Autodesk Inventor part; units mm, degrees
ref_plane "YZ Plane" through (0, 0, 0) normal (1, 0, 0) x (0, 1, 0)
ref_plane "XZ Plane" through (0, 0, 0) normal (0, 1, 0) x (-1, 0, 0)
ref_plane "XY Plane" through (0, 0, 0) normal (0, 0, 1) x (1, 0, 0)
sketch "スケッチ1" plane through (0, 0, 0) normal (0, 0, 1) x (1, 0, 0)
  line L0 (12.35, 15.25) -> (9.34, 15.25)
  line L1 (-15.25, 12.35) -> (-15.25, -12.35)
  line L2 (-12.35, -15.25) -> (-1.66, -15.25)
  line L3 (15.25, -12.35) -> (15.25, 12.35)
  line L4 (-0.66, 6.75) -> (8.34, 6.75)
  line L5 (9.34, 7.75) -> (9.34, 15.25)
  line L6 (-0.66, -6.75) -> (8.34, -6.75)
  line L7 (9.34, -7.75) -> (9.34, -15.25)
  line L8 (9.34, 15.25) -> (-1.66, 15.25) construction
  line L9 (-1.66, 15.25) -> (-12.35, 15.25)
  line L10 (9.34, -15.25) -> (12.35, -15.25)
  line L11 (-1.66, -15.25) -> (9.34, -15.25) construction
  line L12 (-1.66, 15.25) -> (-1.66, 7.75)
  line L13 (-1.66, -15.25) -> (-1.66, -7.75)
  arc A0 (15.25, 12.35) -> (12.35, 15.25) centre (12.35, 12.35) ccw
  arc A1 (12.35, -15.25) -> (15.25, -12.35) centre (12.35, -12.35) ccw
  arc A2 (-15.25, -12.35) -> (-12.35, -15.25) centre (-12.35, -12.35) ccw
  arc A3 (-12.35, 15.25) -> (-15.25, 12.35) centre (-12.35, 12.35) ccw
  arc A4 (-1.66, 7.75) -> (-0.66, 6.75) centre (-0.66, 7.75) ccw
  arc A5 (8.34, 6.75) -> (9.34, 7.75) centre (8.34, 7.75) ccw
  arc A6 (9.34, -7.75) -> (8.34, -6.75) centre (8.34, -7.75) ccw
  arc A7 (-0.66, -6.75) -> (-1.66, -7.75) centre (-0.66, -7.75) ccw
  line L14 (0, 0) -> (0, -35.1049) construction
  line L15 (0, 0) -> (30.4007, 0) construction
  line L16 (3.84, -9) -> (3.84, -1.2529) construction
  arc A8 (15.35, 12.35) -> (12.35, 15.35) centre (12.35, 12.35) ccw construction
  dimension "d0" = 2.9
  dimension "d1" = 1
  dimension "d14" = 8.5
  dimension "d15" = 11
  dimension "d16" = 3.84
  dimension "d17" = 8.5
  dimension "d21" = 3
extrude "押し出し1" add sketch "スケッチ1" along normal blind 4
hole "穴1" at (12.35, 12.35, 0) at (12.35, -12.35, 0) at (-12.35, -12.35, 0) at (-12.35, 12.35, 0) direction (0, 0, 1) diameter 2.1 end through all
chamfer "面取り1" distance 0.25 angle 45 4 edges at (9.34, 15.25, 2) (-1.66, 15.25, 2) (-1.66, -15.25, 2) (9.34, -15.25, 2)
properties part number "QUIKS_SINGLE_COVER"
Source: CAD feature listing. Evaluate the final solid. Frame: model axes, mm. A direction names the side the tool comes from. Coordinates: 2 decimals unless noted, no trailing zeros. Loops run counter-clockwise (first coordinate to the right, second up) from the corner with the lowest first, then second, coordinate; pieces in that order, holes last. Notation, with made-up numbers: M 87,-4.5 L 125,-4.5 A26 ccw 125,16.5 Z; hole C 49.25,-38 d7. An arc over 180 degrees is marked long. Answer in a Markdown table with one row per item.
Q1. Section B-B on x = 2. Return the cut outline in (y, z), plus the area to 3 significant figures.
Answers below:
| item | result |
|---|---|
| outline | M -6.75,0 L 6.75,0 L 6.75,4 L -6.75,4 Z |
| area | 54.0 mm^2 |
Q2. Section A-A on z = 0.6. Return the cut outline in (x, y).
Answers below:
| item | result |
|---|---|
| outline | M -15.25,-12.35 A2.9 ccw -12.35,-15.25 L -1.91,-15.25 L -1.66,-15 L -1.66,-7.75 A1 cw -0.66,-6.75 L 8.34,-6.75 A1 cw 9.34,-7.75 L 9.34,-15 L 9.59,-15.25 L 12.35,-15.25 A2.9 ccw 15.25,-12.35 L 15.25,12.35 A2.9 ccw 12.35,15.25 L 9.59,15.25 L 9.34,15 L 9.34,7.75 A1 cw 8.34,6.75 L -0.66,6.75 A1 cw -1.66,7.75 L -1.66,15 L -1.91,15.25 L -12.35,15.25 A2.9 ccw -15.25,12.35 Z; hole C -12.35,-12.35 d2.1; hole C -12.35,12.35 d2.1; hole C 12.35,-12.35 d2.1; hole C 12.35,12.35 d2.1 |
Q3. Draft query along X for faces 4 (the flat face through (-7, -15.25, 2)), 5 (the flat face through (-15.25, 0, 2)), 6 (the cylindrical face through (12.99, -13.18, 2.03)). Return one class per face: pulls with the +X half, pulls with the -X half, needs draft (parallel to the pull), parting line crosses it, or undercut.
Answers below:
| item | result |
|---|---|
| face 4 | needs draft |
| face 5 | pulls with the -X half |
| face 6 | undercut |
Q4. Set-up query: faces 1 (the cylindrical face through (14.4, 14.4, 2)), 2 (the cylindrical face through (-1.359, 7.035, 1.972)), 3 (the cylindrical face through (9, -7, 2)). Return all of +Z, -Z, +X, -X, +Y, -Y with unobstructed straight access to the full face (end or side cutting, diameter ignored); none if empty.
Answers below:
| item | result |
|---|---|
| face 1 | +Z, -Z, +X, +Y |
| face 2 | +Z, -Z, +Y |
| face 3 | +Z, -Z, -Y |
Q5. First-contact query: pin 1 (2 mm diameter, centred on x = -5, y = 2, fed in from -Z); pin 2 (1.2 mm diameter, centred on x = 5.5, z = 2.5, fed in from -Y). Flat tips, straight axial feed; report the tip coordinate or a pass-through.
Answers below:
| item | result |
|---|---|
| pin 1 | stops at z = 0 |
| pin 2 | stops at y = -6.75 |
Q6. Ray query, probe 1 along X at (y, z) = (-12.35, 1.5); probe 2 along Y at (x, z) = (12.35, 1.7); probe 3 along X at (y, z) = (-11, 1.7). Return the intervals inside material, ascending. Write a range as from..to.
Answers below:
| item | result |
|---|---|
| probe 1 | x = -15.25..-13.4, -11.3..-1.66, 9.34..11.3, 13.4..15.25 |
| probe 2 | y = -15.25..-13.4, -11.3..11.3, 13.4..15.25 |
| probe 3 | x = -15.25..-1.66, 9.34..15.25 |
